Can you work these out from the drawing? Everything is in mm from the part's minimum corner. A direction names the side the tool comes from. Round coordinates to 2 decimals unless told otherwise and drop trailing zeros. Loops run counter-clockwise (first coordinate to the right, second up) from the corner with the lowest first, then second, coordinate; pieces in that order, holes last. Notation, with made-up numbers: M -23,46.25 L 26,46.25 A24 cw 26,77.25 Z; hole C -21.75,24.25 d10. An arc over 180 degrees is marked long. Use a Markdown table: item, result.
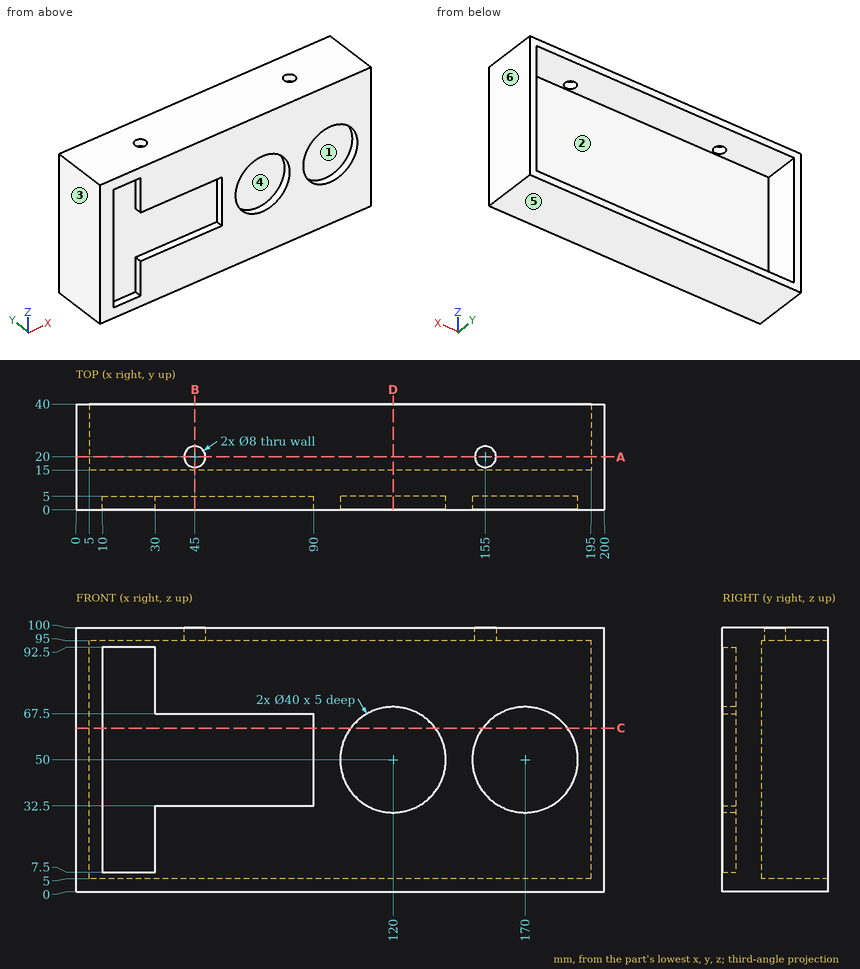
Q1. Imagine slicing it at B-B, the plane x = 45. Please give me the cut outline in (y, z), then the cut area to 4 significant figures.
Return value:
| item | result |
|---|---|
| outline | M 0,0 L 40,0 L 40,5 L 15,5 L 15,95 L 16,95 L 16,100 L 0,100 L 0,67.5 L 5,67.5 L 5,32.5 L 0,32.5 Z; M 24,95 L 40,95 L 40,100 L 24,100 Z |
| area | 1,535 mm^2 |
Q2. Imagine slicing it at A-A, the plane y = 20. Please give me the cut outline in (x, z).
Return value:
| item | result |
|---|---|
| outline | M 0,0 L 200,0 L 200,100 L 159,100 L 159,95 L 195,95 L 195,5 L 5,5 L 5,95 L 41,95 L 41,100 L 0,100 Z; M 49,95 L 151,95 L 151,100 L 49,100 Z |
Q3. Will these pins go through, and if not, where does the flat tip stop? P1, Ø2.5, axis at y = 1.5, z = 17.5, coming from the -X side; P2, Ø5, axis at x = 48.5, z = 80.5, coming from the +Y side; P3, Ø7, axis at x = 155, y = 20, coming from the +Z side.
Return value:
| item | result |
|---|---|
| P1 | stops at x = 0 |
| P2 | stops at y = 15 |
| P3 | stops at z = 5 |
Q4. Imagine slicing it at D-D, the plane x = 120. Please give me the cut outline in (y, z).
Return value:
| item | result |
|---|---|
| outline | M 0,0 L 40,0 L 40,5 L 15,5 L 15,95 L 40,95 L 40,100 L 0,100 L 0,70 L 5,70 L 5,30 L 0,30 Z |
Q5. We'd pull the mould along X, two halves only. Please class the marked faces 4, 5 and 6: pulls with the +X half, pulls with the -X half, needs draft (parallel to the pull), parting line crosses it, or undercut.
Return value:
| item | result |
|---|---|
| face 4 | undercut |
| face 5 | needs draft |
| face 6 | pulls with the +X half |
Q6. I need wall thicknesses on line 1 (Z direction, x = 170, y = 3.25); line 2 (X direction, y = 37.5, z = 49.5); line 3 (Y direction, x = 155, z = 96.6). Which ranges of each line are inside material? Lowest first, please. Write a range as from..to.
Return value:
| item | result |
|---|---|
| line 1 | z = 0..30, 70..100 |
| line 2 | x = 0..5, 195..200 |
| line 3 | y = 0..16, 24..40 |
Q7. For the marked faces 1, 2 and 3, which set-ups out of +Z, -Z, +X, -X, +Y, -Y let a thin tool reach every point of the face, with its end or its side?
Return value:
| item | result |
|---|---|
| face 1 | -Y |
| face 2 | +Y |
| face 3 | +Z, -Z, -X, +Y, -Y |
Q8. Imagine slicing it at C-C, the plane z = 62. Please give me the cut outline in (x, y), then the cut area to 3 significant figures.
Return value:
| item | result |
|---|---|
| outline | M 0,0 L 10,0 L 10,5 L 90,5 L 90,0 L 104,0 L 104,5 L 136,5 L 136,0 L 154,0 L 154,5 L 186,5 L 186,0 L 200,0 L 200,40 L 195,40 L 195,15 L 5,15 L 5,40 L 0,40 Z |
| area | 2,530 mm^2 |
